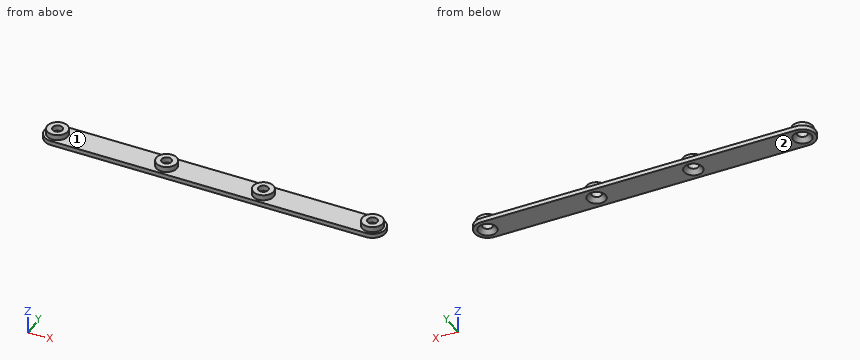
from build123d import *

# Parameters (mm, degrees)
PAD003_DEPTH        = 1.6
SKETCH006_R         = 3.75
PAD004_DEPTH        = 3.6
HOLE001_D           = 3.6
HOLE001_DEPTH       = 25
HOLE001_CSINK_D     = 6.7
HOLE001_CSINK_ANGLE = 90


with BuildPart() as part:
    # Sketch005 → Pad003 (new body)
    with BuildSketch(Plane.XY):
        with BuildLine():
            Line((-57.75, 4.75), (57.75, 4.75))
            ThreePointArc((57.75, -4.75), (62.5, 0), (57.75, 4.75))
            Line((57.75, -4.75), (-57.75, -4.75))
            ThreePointArc((-57.75, 4.75), (-62.5, 0), (-57.75, -4.75))
        make_face()
    extrude(amount=PAD003_DEPTH)

    # Sketch006 → Pad004 (join)
    with BuildSketch(Plane.XY):
        with Locations((-57.75, 0)):
            Circle(SKETCH006_R)
        with Locations((-17.75, 0)):
            Circle(SKETCH006_R)
        with Locations((17.75, 0)):
            Circle(SKETCH006_R)
        with Locations((57.75, 0)):
            Circle(SKETCH006_R)
    extrude(amount=PAD004_DEPTH)

    # Hole001
    with Locations(Plane(origin=(0, 0, 0), x_dir=(1, 0, 0), z_dir=(0, 0, -1))):
        with Locations((-57.75, 0), (-17.75, 0), (17.75, 0), (57.75, 0)):
            CounterSinkHole(HOLE001_D / 2, HOLE001_CSINK_D / 2, depth=HOLE001_DEPTH, counter_sink_angle=HOLE001_CSINK_ANGLE)


with BuildPart() as part_1:
    # Body001 placement: moved
    add(part.part.moved(Location((0, 36, -32))))


solid = part_1.part
For this review, take the finished solid that the model builds, in its own axes (mm). Face numbers are marked on the shaded views. Coordinates: 2 decimals unless noted, no trailing zeros. Write each loop counter-clockwise with the first axis right and the second up, starting at its lowest first coordinate (ties: lowest second). Pieces come first, ordered by that corner, then holes. Notation, with made-up numbers: (0, 68) -> (9, 68) arc R26 ccw to (9, 93) -> close; hole circle Ø6 at (64.5, -32.75). An arc over 180 degrees is marked (long way). Write each question's results on one line, items separated by ' | '. Start each with the question number.
1) Insertion check: pin 1 (1 mm diameter, centred on x = 19.5, z = -29.5, fed in from -Y); pin 2 (4 mm diameter, centred on x = 17.75, y = 36, fed in from -Z); pin 3 (3 mm diameter, centred on x = 57.75, y = 36, fed in from +Z); pin 4 (3 mm diameter, centred on x = -2.5, y = 39.5, fed in from +Z). Each pin has a flat end and moves straight along its axis. Give the tip position at first contact, or say it passes through.
2) Consider section D-D (x = -52). Write out the cut boundary in (y, z), plus the area to 3 significant figures.
3) Consider section A-A (z = -29.7). Write out the cut boundary in (x, y), plus the area to 3 significant figures.
4) Wall thickness on L1, parallel to Y at x = -17.75, z = -28.9; L2, parallel to X at y = 35.75, z = -31.5; L3, parallel to X at y = 35.5, z = -31.7: over which ranges is each line inside the solid? List them lowest first. Write a range as [from, to].
5) The part is to be moulded in two halves that separate along X. For the marked faces 1 and 2, say which applies: +X half, -X half, draft (parallel to the pull), parting line (faces both ways), or undercut.
6) Consider section C-C (y = 36). Give the number of separate pieces and of enclosed holes in the cut face, plus the area to 3 significant figures.
7) Consider section B-B (x = 17.75). Write out the cut boundary in (y, z).
Geometry says:
1) pin 1: y = 32.46 | pin 2: z = -30.65 | pin 3: through | pin 4: z = -30.4
2) outline: (31.25, -32) -> (40.75, -32) -> (40.75, -30.4) -> (31.25, -30.4) -> close | area: 15.2 mm^2
3) outline: circle Ø7.5 at (-57.75, 36); circle Ø7.5 at (-17.75, 36); circle Ø7.5 at (17.75, 36); circle Ø7.5 at (57.75, 36); hole circle Ø3.6 at (-57.75, 36); hole circle Ø3.6 at (-17.75, 36); hole circle Ø3.6 at (17.75, 36); hole circle Ø3.6 at (57.75, 36) | area: 136 mm^2
4) L1: [32.25, 34.2], [37.8, 39.75] | L2: [-62.49, -60.59], [-54.91, -20.59], [-14.91, 14.91], [20.59, 54.91], [60.59, 62.49] | L3: [-62.47, -60.76], [-54.74, -20.76], [-14.74, 14.74], [20.76, 54.74], [60.76, 62.47]
5) face 1: undercut | face 2: draft
6) separate pieces: 5 | enclosed holes: 0 | area: 199 mm^2
7) outline: (31.25, -32) -> (32.65, -32) -> (34.2, -30.45) -> (34.2, -28.4) -> (32.25, -28.4) -> (32.25, -30.4) -> (31.25, -30.4) -> close; (37.8, -30.45) -> (39.35, -32) -> (40.75, -32) -> (40.75, -30.4) -> (39.75, -30.4) -> (39.75, -28.4) -> (37.8, -28.4) -> close
